```python
from build123d import *

# Parameters (mm, degrees)
SKETCH1_R           = 1.5
SKETCH1_R_2         = 3.75
SKETCH1_R_3         = 7.5
SKETCH1_R_4         = 1.45
BOSS_EXTRUDE1_DEPTH = 1.5
FILLET1_R           = 20


with BuildPart() as part:
    # Sketch1 → Boss-Extrude1 (new body, symmetric)
    with BuildSketch(Plane(origin=(0, 0, 0), x_dir=(0, 0, -1), z_dir=(1, 0, 0))):
        with BuildLine():
            ThreePointArc((-6.573033708, 13.483146067), (-14.928995829, -1.457766625), (-3.840572874, -14.5))
            ThreePointArc((-3.840572874, -14.5), (9.14853559, -11.887148378), (15, 0))
            ThreePointArc((15, 0), (7.9499841, 12.71997456), (-6.573033708, 13.483146067))
        make_face()
        with Locations((0, -7)):
            Circle(SKETCH1_R, mode=Mode.SUBTRACT)
        with Locations((-7, 0)):
            Circle(SKETCH1_R, mode=Mode.SUBTRACT)
        Circle(SKETCH1_R_2, mode=Mode.SUBTRACT)
        with Locations((7, 0)):
            Circle(SKETCH1_R, mode=Mode.SUBTRACT)
        with Locations((0, 7)):
            Circle(SKETCH1_R, mode=Mode.SUBTRACT)
        with BuildLine():
            Line((-127.350956164, -7.122008503), (-105, -14.5))
            Line((-105, -14.5), (-3.840572874, -14.5))
            ThreePointArc((-3.840572874, -14.5), (-14.928995829, -1.457766625), (-6.573033708, 13.483146067))
            Line((-6.573033708, 13.483146067), (-25, 4.5))
            Line((-25, 4.5), (-100, 4.5))
            Line((-100, 4.5), (-117.5, 7.5))
            Line((-117.5, 7.5), (-125, 7.5))
            ThreePointArc((-125, 7.5), (-119.696699141, 5.303300859), (-117.5, 0))
            ThreePointArc((-117.5, 0), (-120.605809018, -6.077917869), (-127.350956164, -7.122008503))
        make_face()
        with Locations((-97.5, -5.5)):
            Circle(SKETCH1_R, mode=Mode.SUBTRACT)
        Polygon((-89.5, -6.5), (-89.5, -3.5), (-87.5, -1.5), (-30, -1.5), (-28, -3.5), (-28, -6.5), (-30, -8.5), (-87.5, -8.5), align=None, mode=Mode.SUBTRACT)
        with Locations((-20, -5.5)):
            Circle(SKETCH1_R, mode=Mode.SUBTRACT)
        with Locations((-125, 0)):
            Circle(SKETCH1_R_3)
        with Locations((-125, 0)):
            Circle(SKETCH1_R_4, mode=Mode.SUBTRACT)
    extrude(amount=BOSS_EXTRUDE1_DEPTH, both=True)

    # Fillet1
    fillet1_edges = [part.edges().sort_by_distance(p)[0] for p in [
        (0.75, -14.5, 3.840572874),
        (0, -14.5, 105),
        (0, 7.5, 117.5),
        (0, 4.5, 100),
        (0, 4.5, 25),
    ]]
    fillet(fillet1_edges, radius=FILLET1_R)


solid = part.part
```
Input: part model. Units: mm. Frame: model coordinates. A direction names the side the tool comes from. Round coordinates to 2 decimals unless told otherwise and drop trailing zeros. Loops run counter-clockwise (first coordinate to the right, second up) from the corner with the lowest first, then second, coordinate; pieces in that order, holes last. Notation, with made-up numbers: (63, 47) -> (72, 47) arc R12 cw to (72, 60) -> close; hole circle Ø9 at (-31.75, 26.5). An arc over 180 degrees is marked (long way). Use one line per item in the form item = value. Start each with the question number.
Item 1: Material intervals for L1, parallel to Y at x = 0.85, z = 0; L2, parallel to Z at x = -0.5, y = -0.5; L3, parallel to Y at x = 1.25, z = 47.5, sorted ascending. Write a range as from..to.
Item 2: Contact query for flat-ended pins moving along their axis: pin 1 Ø1.8 at (y, z) = (-5.5, 97.5) entering from -X; pin 2 Ø1.5 at (x, z) = (0.5, 74) entering from -Y; pin 3 Ø0.9 at (x, y) = (-0.5, -5.5) entering from +Z; pin 4 Ø1.5 at (x, y) = (-0.5, -5) entering from -Z. Output: stop coordinate, or through.
Item 3: Mould query, pull axis Y, two halves, no side actions, for faces 5 (the face through (-0.02, 0.07, -5.5)), 6 (the face through (0, 4.5, 63)), 7 (the face through (-0.021, -14.253, 104.915)). Classes: pulls with the +Y half, pulls with the -Y half, needs draft (parallel to the pull), parting line crosses it, or undercut.
Item 4: Section query C-C on z = 0. Return the cut outline in (x, y).
Item 5: Section query A-A on z = 46.5. Return the cut outline in (x, y), then the cut area to 3 significant figures.
Item 6: Set-up query: faces 1 (the face through (0, 7.5, 122)), 2 (the face through (-0.02, 4.57, 99.97)), 3 (the face through (0.02, 1.34, 132.38)), 4 (the face through (0, -1.5, 59)). Return all of +Z, -Z, +X, -X, +Y, -Y with unobstructed straight access to the full face (end or side cutting, diameter ignored); none if empty.
Item 7: Section query D-D on x = -0.1. Count the separate pieces of the cut face and the enclosed holes in it, then the cut area to 3 significant figures.
Item 8: Section query B-B on y = 0. Return the cut outline in (x, z).
Ans:
q1.L1 = -15..-8.5, -5.5..-3.75, 3.75..5.5, 8.5..15
q1.L2 = -14.99..-8.41, -5.59..-3.72, 3.72..5.59, 8.41..123.64, 126.36..132.48
q1.L3 = -14.5..-8.5, -1.5..4.5
q2.pin_1 = through
q2.pin_2 = -14.5
q2.pin_3 = 130.55
q2.pin_4 = -14.39
q3.face_5 = undercut
q3.face_6 = pulls with the +Y half
q3.face_7 = pulls with the -Y half
q4.outline = (-1.5, -15) -> (1.5, -15) -> (1.5, -8.5) -> (-1.5, -8.5) -> close; (-1.5, -5.5) -> (1.5, -5.5) -> (1.5, -3.75) -> (-1.5, -3.75) -> close; (-1.5, 3.75) -> (1.5, 3.75) -> (1.5, 5.5) -> (-1.5, 5.5) -> close; (-1.5, 8.5) -> (1.5, 8.5) -> (1.5, 15) -> (-1.5, 15) -> close
q5.outline = (-1.5, -14.5) -> (1.5, -14.5) -> (1.5, -8.5) -> (-1.5, -8.5) -> close; (-1.5, -1.5) -> (1.5, -1.5) -> (1.5, 4.5) -> (-1.5, 4.5) -> close
q5.area = 36.0 mm^2
q6.face_1 = +Z, +X, -X, +Y
q6.face_2 = +X, -X, +Y
q6.face_3 = +Z, +X, -X
q6.face_4 = +X, -X
q7.separate_pieces = 1
q7.enclosed_holes = 9
q7.area = 2,440 mm^2
q8.outline = (-1.5, -15) -> (1.5, -15) -> (1.5, -8.5) -> (-1.5, -8.5) -> close; (-1.5, -5.5) -> (1.5, -5.5) -> (1.5, -3.75) -> (-1.5, -3.75) -> close; (-1.5, 3.75) -> (1.5, 3.75) -> (1.5, 5.5) -> (-1.5, 5.5) -> close; (-1.5, 8.5) -> (1.5, 8.5) -> (1.5, 123.55) -> (-1.5, 123.55) -> close; (-1.5, 126.45) -> (1.5, 126.45) -> (1.5, 132.5) -> (-1.5, 132.5) -> close
